The model under review builds one solid part; all positions refer to its coordinate system, in mm. Face numbers are marked on the shaded views. A direction names the side the tool comes from. Round coordinates to 2 decimals unless told otherwise and drop trailing zeros. Write each loop counter-clockwise with the first axis right and the second up, starting at its lowest first coordinate (ties: lowest second). Pieces come first, ordered by that corner, then holes. Notation, with made-up numbers: (-17.75, -31) -> (41.25, -31) arc R22 ccw to (41.25, -19) -> close; hole circle Ø8 at (-9, 7). An arc over 180 degrees is marked (long way). Return JSON: item names as keys, results as strings. Group by question number.
1. Tool access review of the marked faces 4 and 5: name each direction out of +Z, -Z, +X, -X, +Y, -Y from which nothing blocks a thin tool from reaching the whole face with its end or side.
2. Take a section at C-C, the plane y = 25. Give the number of separate pieces and of enclosed holes in the cut face, then the cut area to 3 significant figures.
3. Mouldability with a two-part tool opening along Z and no side actions: class the marked faces 1, 2 and 3 as pulls with the +Z half, pulls with the -Z half, needs draft (parallel to the pull), parting line crosses it, or undercut.
4. Clearance check with flat-ended pins moving along their axes: P1, Ø20, axis at y = 16.5, z = -18, coming from the +X side; P2, Ø7.5, axis at x = 72.5, y = 22.5, coming from the +Z side; P3, Ø3, axis at x = -26.5, z = 80, coming from the +Y side. State where each tip first meets the part, or that it passes through.
5. For line 1 along Z through (x, y) = (-43, 16); line 2 along Z through (x, y) = (-30, 22.5); line 3 along X through (y, z) = (15, 4), list the stretches that pass through material, from the lowest coordinate up. Write a range as from..to.
6. Take a section at A-A, the plane z = -52. Write out the cut boundary in (x, y), then the cut area to 3 significant figures.
7. Take a section at B-B, the plane z = 70. Write out the cut boundary in (x, y).
from build123d import *

# Parameters (mm, degrees)
BOSS_EXTRUDE1_DEPTH = 40
BOSS_EXTRUDE1_DRAFT = -15
SHELL1_T            = -10
RIB7_REACH          = 207.359
SKETCH5_WALLS_W     = 5
SKETCH5_WALLS_H     = 549.174801164
SKETCH5_WALLS_W_2   = 496.753269208
SKETCH5_WALLS_H_2   = 5
SKETCH5_WALLS_W_3   = 472.743407243
SKETCH5_WALLS_W_4   = 484.34817386
RIB8_REACH          = 207.359
SKETCH6_WALLS_W     = 5
SKETCH6_WALLS_H     = 444.331737252
RIB9_START          = -2.5
RIB9_DEPTH          = 5


# Read off the part's stored shape, not the designer's step: Rib9
with BuildPart() as part:
    # Sketch1 → Boss-Extrude1 (with draft: the straight prism first)
    with BuildSketch(Plane(origin=(0, 0, 0), x_dir=(1, 0, 0), z_dir=(0, 1, 0))):
        with BuildLine():
            Line((-109.029856613, -113.081906669), (109.029856613, -113.081906669))
            Line((109.029856613, -113.081906669), (109.029856613, 113.081906669))
            ThreePointArc((109.029856613, 113.081906669), (0, 152.401411753), (-109.029856613, 113.081906669))
            Line((-109.029856613, 113.081906669), (-109.029856613, -113.081906669))
        make_face()
    extrude(amount=BOSS_EXTRUDE1_DEPTH)
    # Boss-Extrude1: the draft: its side faces are tilted about the plane it starts from
    boss_extrude1_sides = [part.faces().sort_by_distance(p)[0] for p in [
        (0, 20, 113.081906669),
        (109.029856613, 20, 0),
        (0, 20, -152.401411753),
        (-109.029856613, 20, 0),
    ]]
    draft(boss_extrude1_sides, Plane(origin=(0, 0, 0), x_dir=(1, 0, 0), z_dir=(0, 1, 0)), BOSS_EXTRUDE1_DRAFT)

    # Shell1
    shell1_openings = [part.faces().sort_by_distance(p)[0] for p in [
        (0, 40, -12.878837242),
    ]]
    offset(amount=SHELL1_T, openings=shell1_openings, kind=Kind.INTERSECTION)

    # Sketch5 walls → Rib7 (add, up to next)
    with BuildSketch(Plane(origin=(0, 35, 0), x_dir=(1, 0, 0), z_dir=(0, 1, 0)), mode=Mode.PRIVATE) as rib7_sk1:
        with Locations((0, 17.67893893)):
            Rectangle(SKETCH5_WALLS_W, SKETCH5_WALLS_H)
    rib7_tool1 = extrude(rib7_sk1.sketch, amount=-RIB7_REACH, mode=Mode.PRIVATE) - part.part
    # Sketch5 walls → Rib7 (add, up to next)
    with BuildSketch(Plane(origin=(0, 35, 0), x_dir=(1, 0, 0), z_dir=(0, 1, 0)), mode=Mode.PRIVATE) as rib7_sk2:
        with Locations((6.802794223, -22.557588079)):
            Rectangle(SKETCH5_WALLS_W_2, SKETCH5_WALLS_H_2)
    rib7_tool2 = extrude(rib7_sk2.sketch, amount=-RIB7_REACH, mode=Mode.PRIVATE) - part.part
    # Sketch5 walls → Rib7 (add, up to next)
    with BuildSketch(Plane(origin=(0, 35, 0), x_dir=(1, 0, 0), z_dir=(0, 1, 0)), mode=Mode.PRIVATE) as rib7_sk3:
        with Locations((2.801150562, 37.066902466)):
            Rectangle(SKETCH5_WALLS_W_3, SKETCH5_WALLS_H_2)
    rib7_tool3 = extrude(rib7_sk3.sketch, amount=-RIB7_REACH, mode=Mode.PRIVATE) - part.part
    # Sketch5 walls → Rib7 (add, up to next)
    with BuildSketch(Plane(origin=(0, 35, 0), x_dir=(1, 0, 0), z_dir=(0, 1, 0)), mode=Mode.PRIVATE) as rib7_sk4:
        with Locations((0.600246549, 81.485147101)):
            Rectangle(SKETCH5_WALLS_W_4, SKETCH5_WALLS_H_2)
    rib7_tool4 = extrude(rib7_sk4.sketch, amount=-RIB7_REACH, mode=Mode.PRIVATE) - part.part
    add(rib7_tool1.solids().sort_by_distance((0, 35, -17.67893893))[0])
    add(rib7_tool2.solids().sort_by_distance((6.802794223, 35, 22.557588079))[0])
    add(rib7_tool3.solids().sort_by_distance((2.801150563, 35, -37.066902466))[0])
    add(rib7_tool4.solids().sort_by_distance((0.600246549, 35, -81.485147101))[0])

    # Sketch6 walls → Rib8 (add, up to next)
    with BuildSketch(Plane(origin=(0, 35, 0), x_dir=(1, 0, 0), z_dir=(0, 1, 0)), mode=Mode.PRIVATE) as rib8_sk1:
        with Locations((42.417422804, -59.172627575)):
            Rectangle(SKETCH6_WALLS_W, SKETCH6_WALLS_H)
    rib8_tool1 = extrude(rib8_sk1.sketch, amount=-RIB8_REACH, mode=Mode.PRIVATE) - part.part
    add(rib8_tool1.solids().sort_by_distance((42.417422804, 35, 59.172627575))[0])

    # Rib9 outline → Rib9 (add)
    with BuildSketch(Plane.XY.offset(RIB9_START)):
        Polygon((-74.932871139, 10), (-106.192462318, 28.047733382), (-101.356586733, 10), align=None)
    extrude(amount=RIB9_DEPTH)


solid = part.part
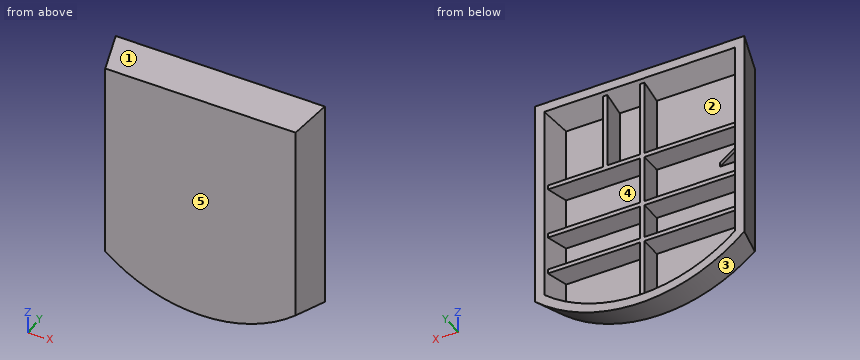
Output:
{
 "1": {"face 4": "+Y", "face 5": "+Z, -Z, +X, -X, -Y"},
 "2": {"separate pieces": "1", "enclosed holes": "9", "area": "14,300 mm^2"},
 "3": {"face 1": "pulls with the +Z half", "face 2": "undercut", "face 3": "pulls with the -Z half"},
 "4": {"P1": "stops at x = 116.13", "P2": "stops at z = 120.12", "P3": "stops at y = 10"},
 "5": {"line 1": "z = -151.33..-140.63, -83.99..-78.99, -39.57..-34.57, 20.06..25.06, 107.02..117.37", "line 2": "z = -155.87..-145.35, -83.99..-78.99, -39.57..-34.57, 20.06..25.06, 108.76..119.11", "line 3": "x = -113.05..-102.7, -2.5..2.5, 102.7..113.05"},
 "6": {"outline": "(-119.75, 40) -> (-109.03, 0) -> (109.03, 0) -> (119.75, 40) -> (109.4, 40) -> (101.36, 10) -> (2.5, 10) -> (2.5, 35) -> (-2.5, 35) -> (-2.5, 10) -> (-101.36, 10) -> (-109.4, 40) -> close", "area": "2,950 mm^2"},
 "7": {"outline": "(-119.75, 40) -> (-109.03, 0) -> (109.03, 0) -> (119.75, 40) -> (109.4, 40) -> (101.36, 10) -> (44.92, 10) -> (44.92, 35) -> (39.92, 35) -> (39.92, 10) -> (2.5, 10) -> (2.5, 35) -> (-2.5, 35) -> (-2.5, 10) -> (-101.36, 10) -> (-109.4, 40) -> close"}
}
